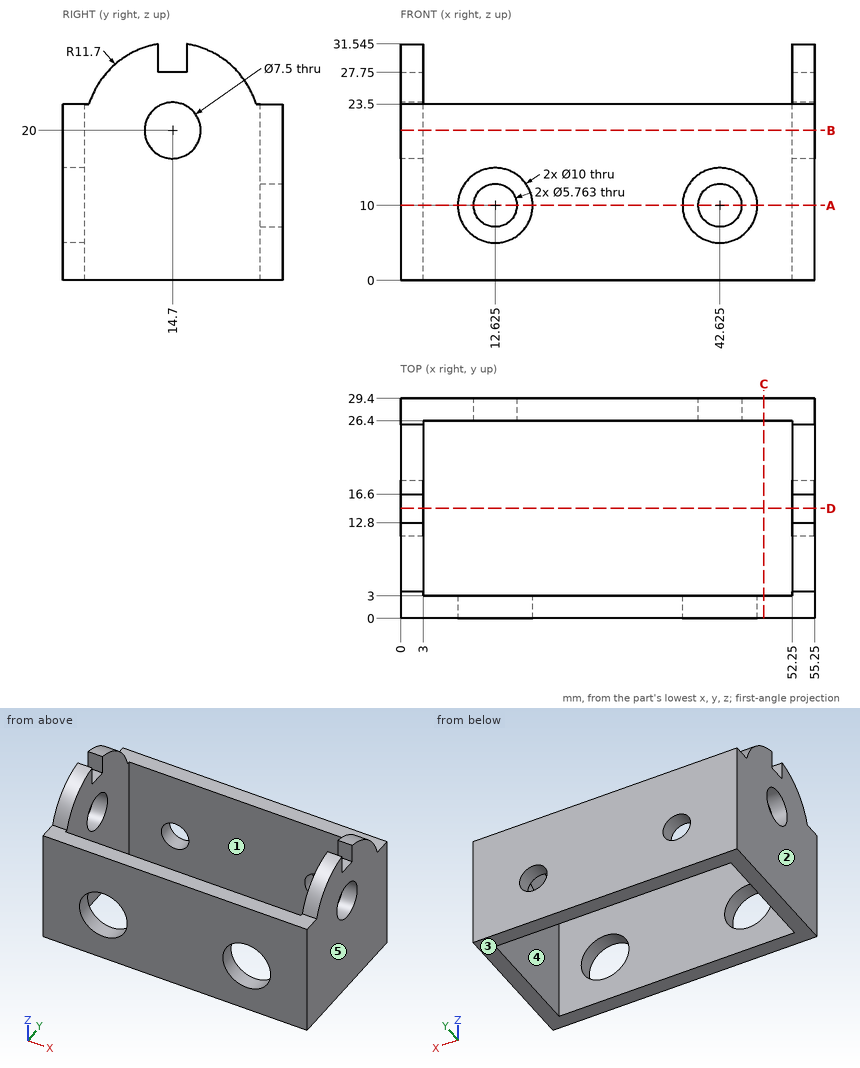
Here's the drawing with two shaded views (mm, measured from the low corner). I have some questions. A direction names the side the tool comes from. Give positions to 0.01 mm unless a question says otherwise; leave off trailing zeros. Order: outer loops, then holes, each group sorted by start corner. A loop starts at its lowest first (then second) coordinate and runs counter-clockwise, first axis right, second up. Notation, with made-up numbers: M 39,25 L 81,25 A17 cw 81,30 Z; hole C 15,10 d11. An arc over 180 degrees is marked long. Answer as a JSON object with one key per item and string values. Group by question number.
1) Suppose I cut it at C-C, the plane x = 48.5. Write out the boundary of the cut face in (y, z), plus the area to 3 significant figures.
2) On a 3-axis mill with a long thin cutter (end or side, diameter ignored), from which of +Z, -Z, +X, -X, +Y, -Y can I reach the whole of each face in a straight line? I mean the marked faces 4 and 5. Say none if no direction works.
3) Please list where these lines run through material, in increasing order: L1, parallel to X at y = 27.3, z = 10; L2, parallel to Y at x = 16.5, z = 3.5; L3, parallel to X at y = 6.5, z = 7.5. Write a range as [from, to].
4) Suppose I cut it at B-B, the plane z = 20. Write out the boundary of the cut face in (x, y).
5) Suppose I cut it at D-D, the plane y = 14.7. Write out the boundary of the cut face in (x, z).
6) We'd pull the mould along X, two halves only. Please class the marked faces 1, 2 and 3: pulls with the +X half, pulls with the -X half, needs draft (parallel to the pull), parting line crosses it, or undercut.
7) I'm going to push flat-ended pins straight in: pin 1 Ø1 at (x, y) = (39.5, 24.5) entering from -Z; pin 2 Ø1.5 at (x, y) = (54.5, 14) entering from +Z; pin 3 Ø2.5 at (x, z) = (53.5, 29) entering from +Y (1 decimal); pin 4 Ø6 at (x, z) = (42.625, 10) entering from -Y. Where does each tip first touch, or does it pass through?
8) Suppose I cut it at A-A, the plane z = 10. Count the separate pieces of the cut face and the enclosed holes in it.
Results found:
{
 "1": {"outline": "M 0,0 L 3,0 L 3,23.5 L 0,23.5 Z; M 26.4,0 L 29.4,0 L 29.4,23.5 L 26.4,23.5 Z", "area": "141 mm²"},
 "2": {"face 4": "+Z, -Z", "face 5": "+Z, -Z, +X, +Y, -Y"},
 "3": {"L1": "[0, 9.74], [15.51, 39.74], [45.51, 55.25]", "L2": "[0, 3], [26.4, 29.4]", "L3": "[0, 3], [52.25, 55.25]"},
 "4": {"outline": "M 0,0 L 55.25,0 L 55.25,10.95 L 52.25,10.95 L 52.25,3 L 3,3 L 3,10.95 L 0,10.95 Z; M 0,18.45 L 3,18.45 L 3,26.4 L 52.25,26.4 L 52.25,18.45 L 55.25,18.45 L 55.25,29.4 L 0,29.4 Z"},
 "5": {"outline": "M 0,0 L 3,0 L 3,16.25 L 0,16.25 Z; M 0,23.75 L 3,23.75 L 3,27.75 L 0,27.75 Z; M 52.25,0 L 55.25,0 L 55.25,16.25 L 52.25,16.25 Z; M 52.25,23.75 L 55.25,23.75 L 55.25,27.75 L 52.25,27.75 Z"},
 "6": {"face 1": "undercut", "face 2": "pulls with the -X half", "face 3": "needs draft"},
 "7": {"pin 1": "through", "pin 2": "z = 27.75", "pin 3": "y = 23.5", "pin 4": "y = 26.4"},
 "8": {"separate pieces": "4", "enclosed holes": "0"}
}
